Here's how the part is built. I have some questions about the finished solid (model axes, mm). Coordinates: 2 decimals unless noted, no trailing zeros. Loops run counter-clockwise (first coordinate to the right, second up) from the corner with the lowest first, then second, coordinate; pieces in that order, holes last. Notation, with made-up numbers: (19.5, -9) -> (37.5, -9) arc R15 ccw to (37.5, 20) -> close; hole circle Ø1 at (88.25, 3.25). An arc over 180 degrees is marked (long way). Answer as a JSON object with one key per item and string values. Group by question number.
Q1. I want a section at D-D on x = 12.5. Write out the boundary of the cut face in (y, z), then the cut area to 3 significant figures.
Q2. I'm going to push flat-ended pins straight in: pin 1 (0.7 mm diameter, centred on x = 31, y = 0.5, fed in from +Z); pin 2 (0.7 mm diameter, centred on y = 0.5, z = 27, fed in from +X); pin 3 (12 mm diameter, centred on x = -5, z = -4, fed in from -Y). Where does each tip first touch, or does it pass through?
Q3. I want a section at C-C on z = 4.5. Write out the boundary of the cut face in (x, y).
Q4. I want a section at B-B on x = -4.5. Write out the boundary of the cut face in (y, z).
Q5. I need wall thicknesses on line 1 (X direction, y = -1.75, z = -3.5); line 2 (Y direction, x = 53, z = -4); line 3 (Y direction, x = -53.2, z = -4.5). Which ranges of each line are inside material? Lowest first, please.
Q6. I want a section at A-A on y = -13. Write out the boundary of the cut face in (x, z).
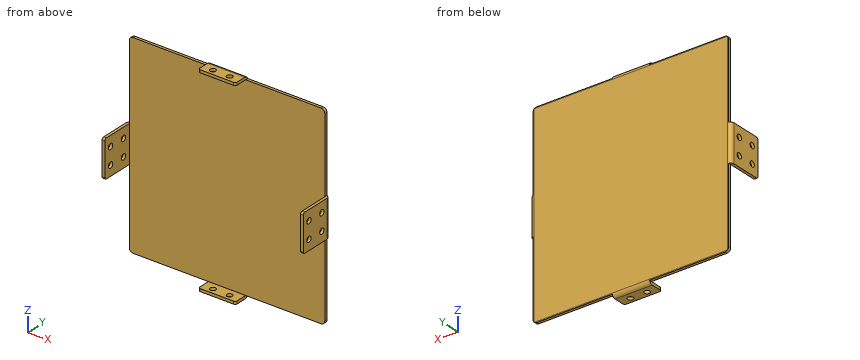
```python
from build123d import *

# Parameters (mm, degrees)
SKETCH1_W           = 105
SKETCH1_H           = 105
BOSS_EXTRUDE1_DEPTH = 1.5
SKETCH2_W           = 20
SKETCH2_H           = 1.5
BOSS_EXTRUDE2_DEPTH = 8.5
SKETCH3_W           = 1.5
SKETCH3_H           = 20
BOSS_EXTRUDE3_DEPTH = 18.45
SKETCH4_R           = 1.5
CUT_EXTRUDE1_DEPTH  = 122.93154842
SKETCH5_R           = 1.5
CUT_EXTRUDE2_DEPTH  = 122.93154842
FILLET1_R           = 1
FILLET2_START       = -53.84589
FILLET2_DEPTH       = 107.69178
FILLET2_START_2     = -53
FILLET2_2_DEPTH     = 106
FILLET3_R           = 2


with BuildPart() as part:
    # Sketch1 → Boss-Extrude1 (new body)
    with BuildSketch(Plane(origin=(0, 0, 0), x_dir=(1, 0, 0), z_dir=(0, 1, 0))):
        Rectangle(SKETCH1_W, SKETCH1_H)
    extrude(amount=BOSS_EXTRUDE1_DEPTH)

    # Sketch2 → Boss-Extrude2 (add)
    with BuildSketch(Plane(origin=(0, 1.5, 0), x_dir=(1, 0, 0), z_dir=(0, 1, 0))):
        with Locations((0, 53.25)):
            Rectangle(SKETCH2_W, SKETCH2_H)
        with Locations((0, -53.25)):
            Rectangle(SKETCH2_W, SKETCH2_H)
    extrude(amount=-BOSS_EXTRUDE2_DEPTH)

    # Sketch3 → Boss-Extrude3 (add)
    with BuildSketch(Plane(origin=(0, 1.5, 0), x_dir=(1, 0, 0), z_dir=(0, 1, 0))):
        with Locations((53.25, 0)):
            Rectangle(SKETCH3_W, SKETCH3_H)
        with Locations((-53.25, 0)):
            Rectangle(SKETCH3_W, SKETCH3_H)
    extrude(amount=-BOSS_EXTRUDE3_DEPTH)

    # Sketch4 → Cut-Extrude1 (cut, through all)
    with BuildSketch(Plane.XY.offset(54)):
        with Locations((-4.5, -4)):
            Circle(SKETCH4_R)
        with Locations(Location((4.5, -4, 0), (0, 0, 180))):
            Circle(SKETCH4_R)
    extrude(amount=-CUT_EXTRUDE1_DEPTH, mode=Mode.SUBTRACT)

    # Sketch5 → Cut-Extrude2 (cut, through all)
    with BuildSketch(Plane(origin=(54, 0, 0), x_dir=(0, 0, -1), z_dir=(1, 0, 0))):
        with Locations((-4.5, -4)):
            Circle(SKETCH5_R)
        with Locations((4.5, -4)):
            Circle(SKETCH5_R)
        with Locations((4.5, -13)):
            Circle(SKETCH5_R)
        with Locations((-4.5, -13)):
            Circle(SKETCH5_R)
    extrude(amount=-CUT_EXTRUDE2_DEPTH, mode=Mode.SUBTRACT)

    # Fillet1
    fillet1_edges = [part.edges().sort_by_distance(p)[0] for p in [
        (-10, -7, -53.25),
        (10, -7, -53.25),
        (-10, -7, 53.25),
        (10, -7, 53.25),
        (53.25, -16.95, -10),
        (53.25, -16.95, 10),
        (-53.25, -16.95, 10),
        (-53.25, -16.95, -10),
    ]]
    fillet(fillet1_edges, radius=FILLET1_R)

    # Fillet2: read off the stored shape, not the designer's step
    # Fillet2 outline → Fillet2 (cut)
    with BuildSketch(Plane.XY.offset(FILLET2_START)):
        with BuildLine():
            ThreePointArc((52, 1.5), (53.414213562, 0.914213562), (54, -0.5))
            Line((54, -0.5), (54, 1.5))
            Line((54, 1.5), (52, 1.5))
        make_face()
        with BuildLine():
            Line((-52, 1.5), (-54, 1.5))
            Line((-54, 1.5), (-54, -0.5))
            ThreePointArc((-54, -0.5), (-53.414213562, 0.914213562), (-52, 1.5))
        make_face()
    extrude(amount=FILLET2_DEPTH, mode=Mode.SUBTRACT)

    # Fillet2 2 outline → Fillet2 2 (cut)
    with BuildSketch(Plane.YZ.offset(FILLET2_START_2)):
        with BuildLine():
            ThreePointArc((1.5, -52), (0.914213562, -53.414213562), (-0.5, -54))
            Line((-0.5, -54), (1.5, -54))
            Line((1.5, -54), (1.5, -52))
        make_face()
        with BuildLine():
            Line((1.5, 52), (1.5, 54))
            Line((1.5, 54), (-0.5, 54))
            ThreePointArc((-0.5, 54), (0.914213562, 53.414213562), (1.5, 52))
        make_face()
    extrude(amount=FILLET2_2_DEPTH, mode=Mode.SUBTRACT)

    # Fillet3
    # the kernel refuses this fillet: 2 mm, written as the material it takes off along each edge
    with BuildSketch(Plane(origin=(52.5, -5, -52.5), x_dir=(0, 0, 1), z_dir=(0, 1, 0)), Plane(origin=(52.5, -5, 52.5), x_dir=(-1, 0, 0), z_dir=(0, 1, 0)), Plane(origin=(-52.5, -5, -52.5), x_dir=(1, 0, 0), z_dir=(0, 1, 0))) as fillet3_piece_1:
        with BuildLine():
            CenterArc((FILLET3_R, -FILLET3_R), FILLET3_R, 90, 90)
            Line((0, -FILLET3_R), (0, 0))
            Line((0, 0), (FILLET3_R, 0))
        make_face()
    extrude(amount=11.436491673, mode=Mode.SUBTRACT)
    with BuildSketch(Plane(origin=(-52.5, -5, 52.5), x_dir=(1, 0, 0), z_dir=(0, 1, 0))) as fillet3_piece_2:
        with BuildLine():
            CenterArc((FILLET3_R, FILLET3_R), FILLET3_R, 180, 90)
            Line((0, FILLET3_R), (0, 0))
            Line((0, 0), (FILLET3_R, 0))
        make_face()
    extrude(amount=11.436491673, mode=Mode.SUBTRACT)


solid = part.part
```
Result set:
{
 "1": {"outline": "(0, -52.5) -> (1.44, -52.5) arc R2 ccw to (1.5, -52) -> (1.5, 52) arc R2 ccw to (1.44, 52.5) -> (0, 52.5) -> close", "area": "157 mm²"},
 "2": {"pin 1": "stops at z = 52.5", "pin 2": "stops at x = 52.5", "pin 3": "stops at y = 0"},
 "3": {"outline": "(-54, -16.95) -> (-52.5, -16.95) -> (-52.5, -14.5) -> (-54, -14.5) -> close; (-54, -11.5) -> (-52.5, -11.5) -> (-52.5, -5.5) -> (-54, -5.5) -> close; (-54, -2.5) -> (-52.5, -2.5) -> (-52.5, 0) -> (52.5, 0) -> (52.5, -2.5) -> (54, -2.5) -> (54, -0.5) arc R2 ccw to (52, 1.5) -> (-52, 1.5) arc R2 ccw to (-54, -0.5) -> close; (52.5, -16.95) -> (54, -16.95) -> (54, -14.5) -> (52.5, -14.5) -> close; (52.5, -11.5) -> (54, -11.5) -> (54, -5.5) -> (52.5, -5.5) -> close"},
 "4": {"outline": "(-7, -54) -> (-5.5, -54) -> (-5.5, -52.5) -> (-7, -52.5) -> close; (-7, 52.5) -> (-5.5, 52.5) -> (-5.5, 54) -> (-7, 54) -> close; (-2.5, -54) -> (-0.5, -54) arc R2 ccw to (1.5, -52) -> (1.5, 52) arc R2 ccw to (-0.5, 54) -> (-2.5, 54) -> (-2.5, 52.5) -> (0, 52.5) -> (0, -52.5) -> (-2.5, -52.5) -> close"},
 "5": {"line 1": "x = -54 to -52.5, 52.5 to 54", "line 2": "y = -16.95 to -14.41, -11.59 to -5.41, -2.59 to 1.23", "line 3": "y = -16.95 to -14.5, -11.5 to -5.5, -2.5 to 1.1"},
 "6": {"outline": "(-54, -10) -> (-52.5, -10) -> (-52.5, -6) -> (-54, -6) -> close; (-54, -3) -> (-52.5, -3) -> (-52.5, 3) -> (-54, 3) -> close; (-54, 6) -> (-52.5, 6) -> (-52.5, 10) -> (-54, 10) -> close; (52.5, -10) -> (54, -10) -> (54, -6) -> (52.5, -6) -> close; (52.5, -3) -> (54, -3) -> (54, 3) -> (52.5, 3) -> close; (52.5, 6) -> (54, 6) -> (54, 10) -> (52.5, 10) -> close"}
}
